Here's how the part is built. I have some questions about the finished solid (model axes, mm). A direction names the side the tool comes from. Round coordinates to 2 decimals unless told otherwise and drop trailing zeros. Loops run counter-clockwise (first coordinate to the right, second up) from the corner with the lowest first, then second, coordinate; pieces in that order, holes last. Notation, with made-up numbers: (18.25, 70.5) -> (56.25, 70.5) arc R25 ccw to (56.25, 101.5) -> close; hole circle Ø10 at (-28, 1.5). An arc over 180 degrees is marked (long way). One line per item, written item: value. Start each with the question number.
```python
from build123d import *

# Parameters (mm, degrees)
SKETCH1_W           = 55.8
SKETCH1_H           = 15.8
BOSS_EXTRUDE1_DEPTH = 28.8
SKETCH2_R           = 7.62
CUT_EXTRUDE1_DEPTH  = 12.7
SKETCH4_R           = 2.778125
SKETCH4_R_2         = 1.8415
CUT_EXTRUDE2_DEPTH  = 12.7
CUT_EXTRUDE6_DEPTH  = 1.905
SKETCH6_R           = 2.425
BOSS_EXTRUDE2_DEPTH = 1.83
SKETCH7_W           = 53.36
SKETCH7_H           = 13.36
SKETCH7_R           = 3.2625
CUT_EXTRUDE7_DEPTH  = 3


with BuildPart() as part:
    # Sketch1 → Boss-Extrude1 (new body)
    with BuildSketch(Plane(origin=(0, 0, 0), x_dir=(1, 0, 0), z_dir=(0, 1, 0))):
        with Locations((-11.199948696, 8.193463303)):
            Rectangle(SKETCH1_W, SKETCH1_H)
    extrude(amount=BOSS_EXTRUDE1_DEPTH)

    # Sketch2 → Cut-Extrude1 (cut)
    with BuildSketch(Plane.XY.offset(-0.293463303)):
        with Locations((0.800051304, 15.4)):
            Circle(SKETCH2_R)
        with BuildLine():
            Line((-11.899948696, 10.6375), (-24.599948696, 10.6375))
            ThreePointArc((-24.599948696, 10.6375), (-29.362448696, 15.4), (-24.599948696, 20.1625))
            Line((-24.599948696, 20.1625), (-11.899948696, 20.1625))
            ThreePointArc((-11.899948696, 20.1625), (-7.137448696, 15.4), (-11.899948696, 10.6375))
        make_face()
    extrude(amount=-CUT_EXTRUDE1_DEPTH, mode=Mode.SUBTRACT)

    # Sketch4 → Cut-Extrude2 (cut)
    with BuildSketch(Plane(origin=(0, 0, -16.093463303), x_dir=(-1, 0, 0), z_dir=(0, 0, -1))):
        with Locations((-0.800051304, 15.4)):
            Circle(SKETCH4_R)
        with Locations((11.899948696, 15.4)):
            Circle(SKETCH4_R_2)
        with Locations((24.599948696, 15.4)):
            Circle(SKETCH4_R_2)
    extrude(amount=-CUT_EXTRUDE2_DEPTH, mode=Mode.SUBTRACT)

    # Sketch5 → Cut-Extrude6 (cut)
    with BuildSketch(Plane(origin=(0, 0, -16.093463303), x_dir=(-1, 0, 0), z_dir=(0, 0, -1))):
        with BuildLine():
            Line((24.599948696, 20.1625), (11.899948696, 20.1625))
            ThreePointArc((11.899948696, 20.1625), (7.137448696, 15.4), (11.899948696, 10.6375))
            Line((11.899948696, 10.6375), (24.599948696, 10.6375))
            ThreePointArc((24.599948696, 10.6375), (29.362448696, 15.4), (24.599948696, 20.1625))
        make_face()
    extrude(amount=-CUT_EXTRUDE6_DEPTH, mode=Mode.SUBTRACT)

    # Sketch6 → Boss-Extrude2 (add)
    with BuildSketch(Plane(origin=(0, 28.8, 0), x_dir=(1, 0, 0), z_dir=(0, 1, 0))):
        with Locations((12.800051304, 12.193463303)):
            Circle(SKETCH6_R)
        with Locations((12.800051304, 4.193463303)):
            Circle(SKETCH6_R)
        with Locations((4.800051304, 12.193463303)):
            Circle(SKETCH6_R)
        with Locations((4.800051304, 4.193463303)):
            Circle(SKETCH6_R)
        with Locations((-3.199948696, 12.193463303)):
            Circle(SKETCH6_R)
        with Locations((-3.199948696, 4.193463303)):
            Circle(SKETCH6_R)
        with Locations((-11.199948696, 12.193463303)):
            Circle(SKETCH6_R)
        with Locations((-11.199948696, 4.193463303)):
            Circle(SKETCH6_R)
        with Locations((-19.199948696, 12.193463303)):
            Circle(SKETCH6_R)
        with Locations((-19.199948696, 4.193463303)):
            Circle(SKETCH6_R)
        with Locations((-27.199948696, 12.193463303)):
            Circle(SKETCH6_R)
        with Locations((-27.199948696, 4.193463303)):
            Circle(SKETCH6_R)
        with Locations((-35.199948696, 12.193463303)):
            Circle(SKETCH6_R)
        with Locations((-35.199948696, 4.193463303)):
            Circle(SKETCH6_R)
    extrude(amount=BOSS_EXTRUDE2_DEPTH)

    # Sketch7 → Cut-Extrude7 (cut)
    with BuildSketch(Plane.XZ):
        with Locations((-11.199948696, -8.193463303)):
            Rectangle(SKETCH7_W, SKETCH7_H)
        with Locations((8.800051304, -8.193463303)):
            Circle(SKETCH7_R, mode=Mode.SUBTRACT)
        with Locations((0.800051304, -8.193463303)):
            Circle(SKETCH7_R, mode=Mode.SUBTRACT)
        with Locations((-7.199948696, -8.193463303)):
            Circle(SKETCH7_R, mode=Mode.SUBTRACT)
        with Locations((-15.199948696, -8.193463303)):
            Circle(SKETCH7_R, mode=Mode.SUBTRACT)
        with Locations((-23.199948696, -8.193463303)):
            Circle(SKETCH7_R, mode=Mode.SUBTRACT)
        with Locations((-31.199948696, -8.193463303)):
            Circle(SKETCH7_R, mode=Mode.SUBTRACT)
    extrude(amount=-CUT_EXTRUDE7_DEPTH, mode=Mode.SUBTRACT)


solid = part.part
```
Q1. Will these pins go through, and if not, where does the flat tip stop? P1, Ø3, axis at x = -24.6, y = 15.4, coming from the +Z side; P2, Ø5, axis at x = -19, y = 17.5, coming from the -Z side; P3, Ø2, axis at x = -20, z = -15, coming from the +Y side; P4, Ø7.5, axis at x = 2, y = 13.5, coming from the +Z side.
Q2. I want a section at B-B on y = 21. Please give me the cut outline in (x, z).
Q3. I want a section at C-C on z = -3.5. State how many separate pieces and enclosed holes the cut face has, plus the area to 3 significant figures.
Q4. If I drill on line 1 along X through (y, z) = (13, -0.75); line 2 along Y through (x, z) = (-19.5, -10); line 3 along X through (y, z) = (12, -9), over which ranges is the centre line in solid material (lowest first)?
Q5. I want a section at A-A on y = 15.4. Please give me the cut outline in (x, z).
Q6. If we mould it in two halves opening along Z, with no side actions, what happens to faces 5 (the flat face through (1, 12, -12.993)), 6 (the flat face through (-35, 30.63, -12)), 7 (the cylindrical face through (2.377, 29.702, -4.3))? For each: released by +Z, released by -Z, zero draft, split by the parting line, or undercut.
Q7. Which directions (+Z, -Z, +X, -X, +Y, -Y) give clear straight access to the entire face, cutting with the end or side of a thin tool? Please do faces 1 (the cylindrical face through (-29.36, 15.3, -6.55)), 2 (the flat face through (-37.88, 1, -8)), 3 (the cylindrical face through (-29.36, 15.3, -15.15)), 4 (the flat face through (1, 0, -8)).
Answers below:
1. P1: passes through
1. P2: stops at z = -14.19
1. P3: stops at y = 30.63
1. P4: stops at z = -12.99
2. outline: (-39.1, -16.09) -> (16.7, -16.09) -> (16.7, -0.29) -> (5.97, -0.29) -> (5.97, -12.99) -> (-4.37, -12.99) -> (-4.37, -0.29) -> (-39.1, -0.29) -> close
3. separate pieces: 1
3. enclosed holes: 2
3. area: 1,130 mm^2
4. line 1: x = -39.1 to -28.71, -7.79 to -6.43, 8.03 to 16.7
4. line 2: y = 3 to 10.64, 20.16 to 30.63
4. line 3: x = -39.1 to -27.93, -8.57 to -6.02, 7.62 to 16.7
5. outline: (-39.1, -16.09) -> (-29.36, -16.09) -> (-29.36, -14.19) -> (-26.44, -14.19) -> (-26.44, -12.99) -> (-29.36, -12.99) -> (-29.36, -0.29) -> (-39.1, -0.29) -> close; (-22.76, -14.19) -> (-13.74, -14.19) -> (-13.74, -12.99) -> (-22.76, -12.99) -> close; (-10.06, -14.19) -> (-7.14, -14.19) -> (-7.14, -16.09) -> (-1.98, -16.09) -> (-1.98, -12.99) -> (-6.82, -12.99) -> (-6.82, -0.29) -> (-7.14, -0.29) -> (-7.14, -12.99) -> (-10.06, -12.99) -> close; (3.58, -16.09) -> (16.7, -16.09) -> (16.7, -0.29) -> (8.42, -0.29) -> (8.42, -12.99) -> (3.58, -12.99) -> close
6. face 5: released by +Z
6. face 6: zero draft
6. face 7: undercut
7. face 1: +Z
7. face 2: -Y
7. face 3: -Z
7. face 4: +Z, -Z, +X, -X, -Y
